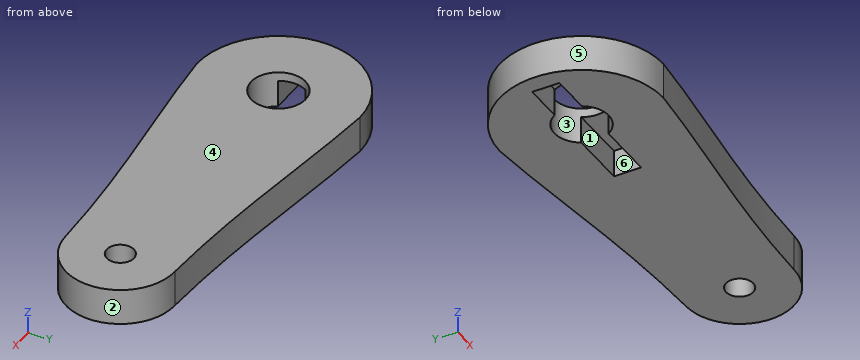
from build123d import *

# Parameters (mm, degrees)
SKETCH_1_R          = 3
SKETCH_1_R_2        = 1.5
EXTRUDE_1_DEPTH     = 4
CUT_EXTRUDE_1_DEPTH = 3


with BuildPart() as part:
    # 草图1 → 凸台-拉伸1 (new body)
    with BuildSketch(Plane.XY):
        with BuildLine():
            ThreePointArc((0, 9), (-9, 0), (0, -9))
            add(Edge.make_bspline(
                [(0, -9), (10.112579717, -8.18843742), (18.689885647, -6.328249505), (30.93, -6)],
                knots=[0, 0, 0, 0, 1, 1, 1, 1], degree=3))
            ThreePointArc((30.93, -6), (36.93, 0), (30.93, 6))
            add(Edge.make_bspline(
                [(0, 9), (10.112579717, 8.18843742), (18.689885647, 6.328249505), (30.93, 6)],
                knots=[0, 0, 0, 0, 1, 1, 1, 1], degree=3))
        make_face()
        Circle(SKETCH_1_R, mode=Mode.SUBTRACT)
        with Locations((30.93, 0)):
            Circle(SKETCH_1_R_2, mode=Mode.SUBTRACT)
    extrude(amount=EXTRUDE_1_DEPTH)

    # 草图2 → 切除-拉伸1 (cut)
    with BuildSketch(Plane.XY):
        Polygon((-2.598076211, 1.5), (-7, 1.5), (-7, -1.5), (9, -1.5), (9, 1.5), align=None)
    extrude(amount=CUT_EXTRUDE_1_DEPTH, mode=Mode.SUBTRACT)


solid = part.part
Geometry check sheet. Reference: the model listing, model coordinates, mm. Face numbers are marked on the shaded views. A direction names the side the tool comes from. Give positions to 0.01 mm unless a question says otherwise; leave off trailing zeros. Loops run counter-clockwise (first coordinate to the right, second up) from the corner with the lowest first, then second, coordinate; pieces in that order, holes last.
(1) Section check C-C on z = 1.4. Count the separate pieces of the cut face and the enclosed holes in it, then the cut area to 3 significant figures.
From the geometry:
separate pieces: 1
enclosed holes: 2
area: 571 mm2
(2) Thickness scan on L1, parallel to Y at x = 30.93, z = 3.05; L2, parallel to Y at x = 3, z = 2.3; L3, parallel to X at y = -2.75, z = 1. Record the ranges inside material, lowest first.
From the geometry:
L1: y = -6 to -1.5, 1.5 to 6
L2: y = -8.73 to -1.5, 1.5 to 8.73
L3: x = -8.57 to -1.2, 1.2 to 36.26
(3) Section check A-A on y = 0. Record the cut outline in (x, z), then the cut area to 3 significant figures.
From the geometry:
outline: (-9, 0) - (-7, 0) - (-7, 3) - (-3, 3) - (-3, 4) - (-9, 4) - close; (3, 3) - (9, 3) - (9, 0) - (29.43, 0) - (29.43, 4) - (3, 4) - close; (32.43, 0) - (36.93, 0) - (36.93, 4) - (32.43, 4) - close
area: 118 mm2
(4) Section check D-D on y = 5. Record the cut outline in (x, z).
From the geometry:
outline: (-7.48, 0) - (34.25, 0) - (34.25, 4) - (-7.48, 4) - close
(5) Set-up check for the marked faces 1 and 2: record each of +Z, -Z, +X, -X, +Y, -Y from which the full face is reachable in a straight line by a thin tool's end or side.
From the geometry:
face 1: -Z
face 2: +Z, -Z, +X
(6) Depth check by flat-ended pin: pin 1 Ø1.8 at (x, y) = (30.93, 0) entering from -Z. Enter the tip coordinate at first touch or a pass-through.
From the geometry:
pin 1: passes through
(7) Section check B-B on y = -2.5. Record the cut outline in (x, z).
From the geometry:
outline: (-8.65, 0) - (-1.66, 0) - (-1.66, 4) - (-8.65, 4) - close; (1.66, 0) - (36.38, 0) - (36.38, 4) - (1.66, 4) - close
(8) Release check for a two-part mould opening along Y. For the marked faces 3, 4, 5 and 6 record: released by +Y, released by -Y, zero draft, split by the parting line, or undercut.
From the geometry:
face 3: undercut
face 4: zero draft
face 5: split by the parting line
face 6: undercut
